Autodesk Fusion 360 part; units mm, degrees
sketch "スケッチ1" plane through (0, 0, 0) normal (0, 0, 1) x (1, 0, 0)
  line L0 (2.5, 186) -> (-92.5, 186)
  line L1 (-92.5, 186) -> (-92.5, -186)
  line L2 (-92.5, -186) -> (2.5, -186)
  line L3 (92.5, 20) -> (92.5, 180)
  line L4 (89.5161, 180) -> (-92.5, -186) construction
  line L5 (-92.5, 186) -> (46.8836, -94.274) construction
  line L6 (2.5, 186) -> (2.5, 180)
  line L7 (2.5, 180) -> (92.5, 180)
  line L8 (-92.5, -186) -> (2.5, -186) construction
  line L9 (92.5, 0) -> (2.5, -186)
  line L10 (92.5, 0) -> (2.5, 0)
  line L11 (2.5, 0) -> (2.5, 20)
  line L12 (2.5, 20) -> (92.5, 20)
  dimension "d2" = 372
  dimension "d5" = 95
  dimension "d15" = 90
  dimension "d16" = 20
extrude "押し出し1" add sketch "スケッチ1" along normal blind 6
chamfer "面取り1" distance 30 angle 45 2 edges at (-92.5, -186, 3) (-92.5, 186, 3)
sketch "スケッチ2" plane through (0, 0, 6) normal (0, 0, 1) x (-1, 0, 0)
  line L0 (62.5, -186) -> (92.5, -156)
  line L1 (92.5, -156) -> (92.5, 156)
  line L2 (92.5, 156) -> (62.5, 186)
  line L3 (62.5, 186) -> (-2.5, 186)
  line L4 (-2.5, 186) -> (-92.5, 0)
  line L5 (-92.5, -20) -> (-92.5, -180)
  line L6 (-92.5, -180) -> (-2.5, -180)
  line L7 (-2.5, -180) -> (-2.5, -186)
  line L8 (-2.5, -186) -> (62.5, -186)
  line L9 (-92.5, -180) -> (-52.5, -180) construction
  line L10 (-52.5, -180) -> (-52.5, -130) construction
  line L11 (-52.5, -130) -> (-92.5, -130) construction
  line L12 (-92.5, -130) -> (-92.5, -180) construction
  line L13 (-52.5, -130) -> (-52.5, -70) construction
  line L14 (-92.5, 0) -> (-2.5, 0)
  line L15 (-2.5, 0) -> (-2.5, -20)
  line L16 (-2.5, -20) -> (-92.5, -20)
  point P0 (-52.5, -130)
  point P1 (-52.5, -70)
  dimension "d10" = 40
  dimension "d11" = 50
  dimension "d12" = 60
hole "穴1" at (52.5, 130, 6) at (52.5, 70, 6) direction (0, 0, -1) diameter 18 end through all
equation "d5 = 30 mm + 65 mm"
The listing builds one solid part. Answer for the finished solid, in the listing's coordinates (mm). Coordinates: 2 decimals unless noted, no trailing zeros. Write each loop counter-clockwise with the first axis right and the second up, starting at its lowest first coordinate (ties: lowest second). Pieces come first, ordered by that corner, then holes. Notation, with made-up numbers: (30.25, 12) - (65.25, 12) arc R23 ccw to (65.25, 39) - close; hole circle Ø7 at (-25.5, -37). An arc over 180 degrees is marked (long way). Put each result on its own line as item: value.
1. The part is cut by section A-A on y = 70. Give the vertices of the cut face in (x, z), plus the area to 3 significant figures.
Answer sheet:
outline: (-92.5, 0) - (43.5, 0) - (43.5, 6) - (-92.5, 6) - close; (61.5, 0) - (92.5, 0) - (92.5, 6) - (61.5, 6) - close
area: 1,000 mm^2
2. Flat-ended cylindrical pins translate along their axes: pin 1 Ø1.8 at (y, z) = (184, 3.5) entering from +X; pin 2 Ø3 at (x, z) = (25.5, 3) entering from -Y. Find the tip coordinate at first contact, or state that the pin passes through.
Answer sheet:
pin 1: stops at x = 2.5
pin 2: stops at y = -141.57
3. The part is cut by section C-C on x = 52.5. Give the vertices of the cut face in (y, z), plus the area to 3 significant figures.
Answer sheet:
outline: (-82.67, 0) - (0, 0) - (0, 6) - (-82.67, 6) - close; (20, 0) - (61, 0) - (61, 6) - (20, 6) - close; (79, 0) - (121, 0) - (121, 6) - (79, 6) - close; (139, 0) - (180, 0) - (180, 6) - (139, 6) - close
area: 1,240 mm^2
4. The part is cut by section D-D on y = -80. Give the vertices of the cut face in (x, z), plus the area to 3 significant figures.
Answer sheet:
outline: (-92.5, 0) - (53.79, 0) - (53.79, 6) - (-92.5, 6) - close
area: 878 mm^2
5. The part is cut by section B-B on z = 3.05. Give the vertices of the cut face in (x, y), plus the area to 3 significant figures.
Answer sheet:
outline: (-92.5, -156) - (-62.5, -186) - (2.5, -186) - (92.5, 0) - (2.5, 0) - (2.5, 20) - (92.5, 20) - (92.5, 180) - (2.5, 180) - (2.5, 186) - (-62.5, 186) - (-92.5, 156) - close; hole circle Ø18 at (52.5, 70); hole circle Ø18 at (52.5, 130)
area: 56,700 mm^2
6. Determine the mould class of faces 1 (the face through (-77.7, -170.8, 3)), 2 (the face through (-77.3, 171.2, 3)), 3 (the face through (49.797, 61.416, 2.958)) for opening direction Y: pulls with the +Y half, pulls with the -Y half, needs draft (parallel to the pull), parting line crosses it, or undercut.
Answer sheet:
face 1: pulls with the -Y half
face 2: pulls with the +Y half
face 3: undercut
7. Find the intervals of material crossed by line 1 along X through (y, z) = (70, 4.25); line 2 along Y through (x, z) = (52.5, 2); line 3 along Y through (x, z) = (77.5, 3.6), in increasing order. Write a range as from..to.
Answer sheet:
line 1: x = -92.5..43.5, 61.5..92.5
line 2: y = -82.67..0, 20..61, 79..121, 139..180
line 3: y = -31..0, 20..180
